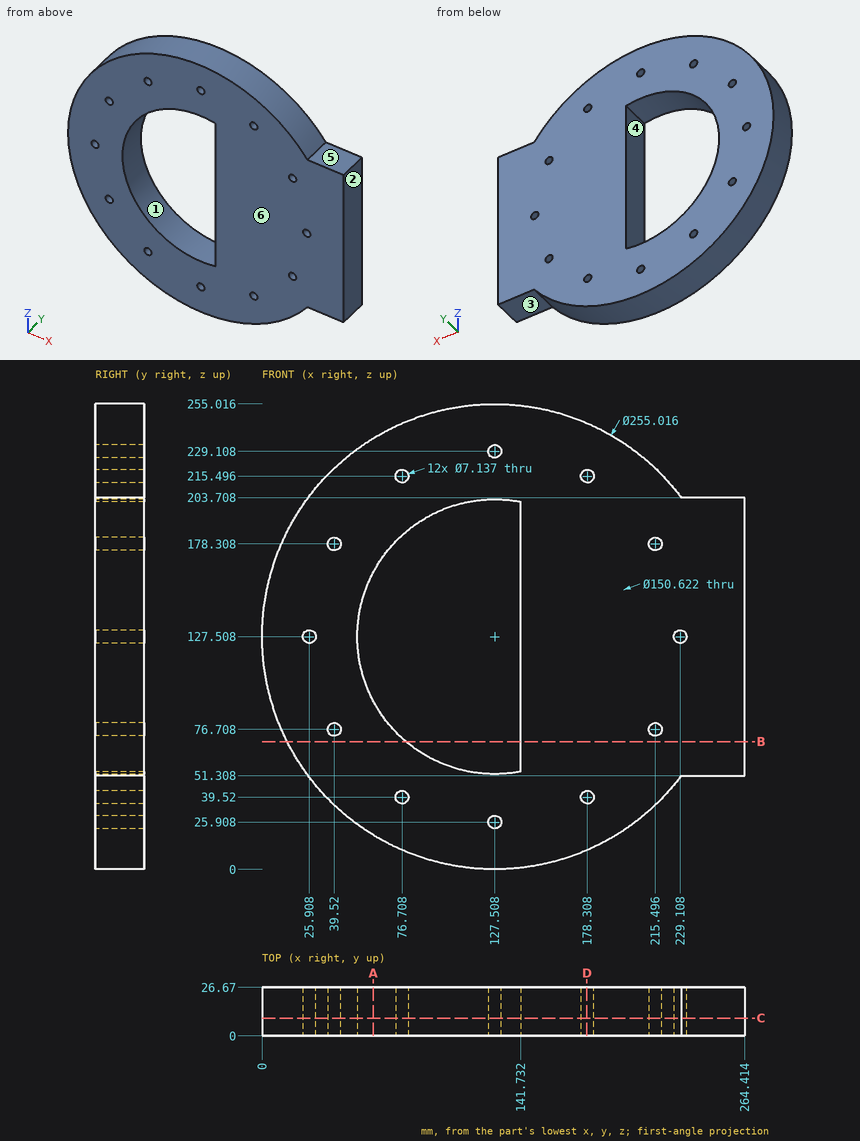
For this review, use the dimensioned drawing (mm, ordinates from the lowest corner) and the shaded views. A direction names the side the tool comes from. Round coordinates to 2 decimals unless told otherwise and drop trailing zeros. Write each loop counter-clockwise with the first axis right and the second up, starting at its lowest first coordinate (ties: lowest second). Pieces come first, ordered by that corner, then holes. Notation, with made-up numbers: (-9.5, 49.5) - (17.5, 49.5) arc R20 ccw to (17.5, 72.5) - close; hole circle Ø3 at (25, 19.25). An arc over 180 degrees is marked (long way). Use CSV: the item, a comma, the result in double quotes.
1) For the marked faces 4, 5 and 6, list the 3-axis set-ups (+Z, -Z, +X, -X, +Y, -Y) from which the entire face can be reached by the end or side of a thin tool; tool diameter is ignored.
Conclusion:
face 4,"+Y, -Y"
face 5,"+Z, +X, +Y, -Y"
face 6,"+Z, -Z, +X, -X, -Y"
2) Clearance check with flat-ended pins moving along their axes: pin 1 Ø5.5 at (x, z) = (76.71, 39.52) entering from -Y; pin 2 Ø2 at (x, y) = (164.5, 16) entering from +Z; pin 3 Ø2 at (x, y) = (133.5, 17) entering from +Z; pin 4 Ø10 at (x, y) = (86.5, 23) entering from -Z. State where each tip first meets the part, or that it passes through.
Conclusion:
pin 1,"passes through"
pin 2,"stops at z = 249.83"
pin 3,"stops at z = 254.92"
pin 4,"stops at z = 5.19"
3) Add section C-C on y = 9.75. Count the separate pieces of the cut face and the enclosed holes in it, and give its area (3 significant figures).
Conclusion:
separate pieces,"1"
enclosed holes,"13"
area,"42,200 mm^2"
4) The part is to be moulded in two halves that separate along X. For the marked faces 1, 2 and 3, say which applies: pulls with the +X half, pulls with the -X half, needs draft (parallel to the pull), parting line crosses it, or undercut.
Conclusion:
face 1,"undercut"
face 2,"pulls with the +X half"
face 3,"needs draft"
5) Add section D-D on x = 178. Write out the cut boundary in (y, z) (1 decimal), and give its area (3 significant figures).
Conclusion:
outline,"(0, 10.4) - (26.7, 10.4) - (26.7, 36) - (0, 36) - close; (0, 43.1) - (26.7, 43.1) - (26.7, 211.9) - (0, 211.9) - close; (0, 219.1) - (26.7, 219.1) - (26.7, 244.6) - (0, 244.6) - close"
area,"5,870 mm^2"
6) Add section B-B on z = 70. Write out the cut boundary in (x, y) (1 decimal).
Conclusion:
outline,"(13.7, 0) - (78.9, 0) - (78.9, 26.7) - (13.7, 26.7) - close; (141.7, 0) - (264.4, 0) - (264.4, 26.7) - (141.7, 26.7) - close"
7) Wall thickness on line 1 along X through (y, z) = (6.25, 74) (1 decimal); line 2 along Z through (x, y) = (39.5, 4) (1 decimal); line 3 along Z through (x, y) = (179, 20.5) (1 decimal): over which ranges is each line inside the solid? List them lowest first. Write a range as from..to.
Conclusion:
line 1,"x = 11.8..37.2, 41.8..74.5, 141.7..213.2, 217.8..264.4"
line 2,"z = 35.2..73.1, 80.3..174.7, 181.9..219.8"
line 3,"z = 10.9..36, 43..212, 219..244.2"
8) Add section A-A on x = 61. Write out the cut boundary in (y, z) (1 decimal), and give its area (3 significant figures).
Conclusion:
outline,"(0, 18.7) - (26.7, 18.7) - (26.7, 92.2) - (0, 92.2) - close; (0, 162.8) - (26.7, 162.8) - (26.7, 236.3) - (0, 236.3) - close"
area,"3,920 mm^2"
